Autodesk Inventor part; units mm, degrees
ref_plane "YZ Plane" through (0, 0, 0) normal (1, 0, 0) x (0, 1, 0)
ref_plane "XZ Plane" through (0, 0, 0) normal (0, 1, 0) x (-1, 0, 0)
ref_plane "XY Plane" through (0, 0, 0) normal (0, 0, 1) x (1, 0, 0)
sketch "Sketch1" plane through (0, 0, 0) normal (0, 1, 0) x (-1, 0, 0)
  line L0 (0, 0) -> (0, 67)
  line L1 (0, 67) -> (67, 67)
  line L2 (67, 64) -> (3, 64)
  line L3 (3, 64) -> (3, 0)
  line L4 (67, 67) -> (67, 64)
  line L5 (3, 0) -> (0, 0)
  dimension "d0" = 67
  dimension "d1" = 67
  dimension "d2" = 3
extrude "Extrusion1" add sketch "Sketch1" along normal blind 20
sketch "Sketch2" plane through (-3, 0, 64) normal (0, 0, -1) x (-1, 0, 0)
  line L0 (64, 0) -> (64, 20) construction
  line L1 (64, 10) -> (0, 10) construction
  line L2 (0, 0) -> (0, 20) construction
  circle A0 centre (50.5, 10) radius 2.65
  circle A1 centre (18.7, 10) radius 2.65
  point P0 (-3, 0)
  dimension "d5" = 5.3
  dimension "d6" = 5.3
  dimension "d7" = 13.5
  dimension "d8" = 31.8
extrude "Extrusion2" cut sketch "Sketch2" against normal up to next
sketch "Sketch3" plane through (-3, 0, 0) normal (-1, 0, 0) x (0, 0, 1)
  line L0 (0, 0) -> (0, 20) construction
  line L1 (0, 10) -> (64, 10) construction
  line L2 (64, 0) -> (64, 20) construction
  circle A0 centre (13.5, 10) radius 2.65
  circle A1 centre (45.3, 10) radius 2.65
  dimension "d11" = 5.3
  dimension "d12" = 5.3
  dimension "d13" = 13.5
  dimension "d14" = 31.8
extrude "Extrusion3" cut sketch "Sketch3" against normal up to next
chamfer "Chamfer1" distance 2 angle 45 4 edges at (-50.85, 10, 64) (-19.05, 10, 64) (-3, 10, 42.65) (-3, 10, 10.85)
chamfer "Chamfer2" distance 6 angle 45 4 edges at (-67, 0, 65.5) (-67, 20, 65.5) (-1.5, 0, 0) (-1.5, 20, 0)
fillet "Fillet1" radius 3 1 edges at (0, 10, 67)
equation "\"d1\" = d0"
equation "\"d6\" = d5"
equation "\"d12\" = d11"
properties part number "90 deg Shelf 4 Hole Bracket"
For this review, take the finished solid that the model builds, in its own axes (mm). A direction names the side the tool comes from. Round coordinates to 2 decimals unless told otherwise and drop trailing zeros. Write each loop counter-clockwise with the first axis right and the second up, starting at its lowest first coordinate (ties: lowest second). Pieces come first, ordered by that corner, then holes.
1) Take a section at B-B on x = -21.7. Give the boundary of the cut face in (y, z).
Answer below:
outline: (0, 64) - (5.35, 64) - (7.35, 66) - (7.35, 67) - (0, 67) - close; (12.65, 66) - (14.65, 64) - (20, 64) - (20, 67) - (12.65, 67) - close
2) Take a section at D-D on y = 17. Give the boundary of the cut face in (x, z).
Answer below:
outline: (-64, 64) - (-3, 64) - (-3, 3) - (0, 3) - (0, 64) arc R3 ccw to (-3, 67) - (-64, 67) - close
3) Mouldability with a two-part tool opening along Y and no side actions: class faces 1 (the face through (0, 10, 32)), 2 (the face through (-64, 17, 66)), 3 (the face through (-55.95, 8.99, 66.49)), 4 (the face through (-21.098, 7.291, 65.875)) as +Y half, -Y half, draft (parallel to the pull), parting line (faces both ways), or undercut.
Answer below:
face 1: draft
face 2: +Y half
face 3: undercut
face 4: undercut
4) Take a section at C-C on z = 45.3. Give the boundary of the cut face in (x, y), then the cut area to 3 significant figures.
Answer below:
outline: (-3, 0) - (0, 0) - (0, 7.35) - (-1, 7.35) - (-3, 5.35) - close; (-3, 14.65) - (-1, 12.65) - (0, 12.65) - (0, 20) - (-3, 20) - close
area: 40.1 mm2
5) Take a section at A-A on y = 10. State how many separate pieces and enclosed holes the cut face has, then the cut area to 3 significant figures.
Answer below:
separate pieces: 5
enclosed holes: 0
area: 311 mm2
6) Insertion check: pin 1 Ø3 at (y, z) = (10, 45.3) entering from -X; pin 2 Ø2 at (y, z) = (14, 10.5) entering from -X; pin 3 Ø4 at (x, y) = (-27, 18) entering from -Z. Each pin has a flat end and moves straight along its axis. Give the tip position at first contact, or say it passes through.
Answer below:
pin 1: passes through
pin 2: stops at x = -3
pin 3: stops at z = 64
7) For line 1 along Y through (x, z) = (-0.75, 45.3); line 2 along X through (y, z) = (6, 54); line 3 along Z through (x, y) = (-4.5, 1), list the stretches that pass through material, from the lowest coordinate up.
Answer below:
line 1: y = 0 to 7.35, 12.65 to 20
line 2: x = -3 to 0
line 3: z = 64 to 67
8) Machinability: for faces 5 (the face through (-1, 0, 50)), 6 (the face through (-3, 10, 32)), which of the approach directions +Z, -Z, +X, -X, +Y, -Y give a long, thin tool a straight path to every point of the face, cutting with its end or side? Answer none if there is none.
Answer below:
face 5: +Z, -Z, +X, -X, -Y
face 6: -Z, -X, +Y, -Y
